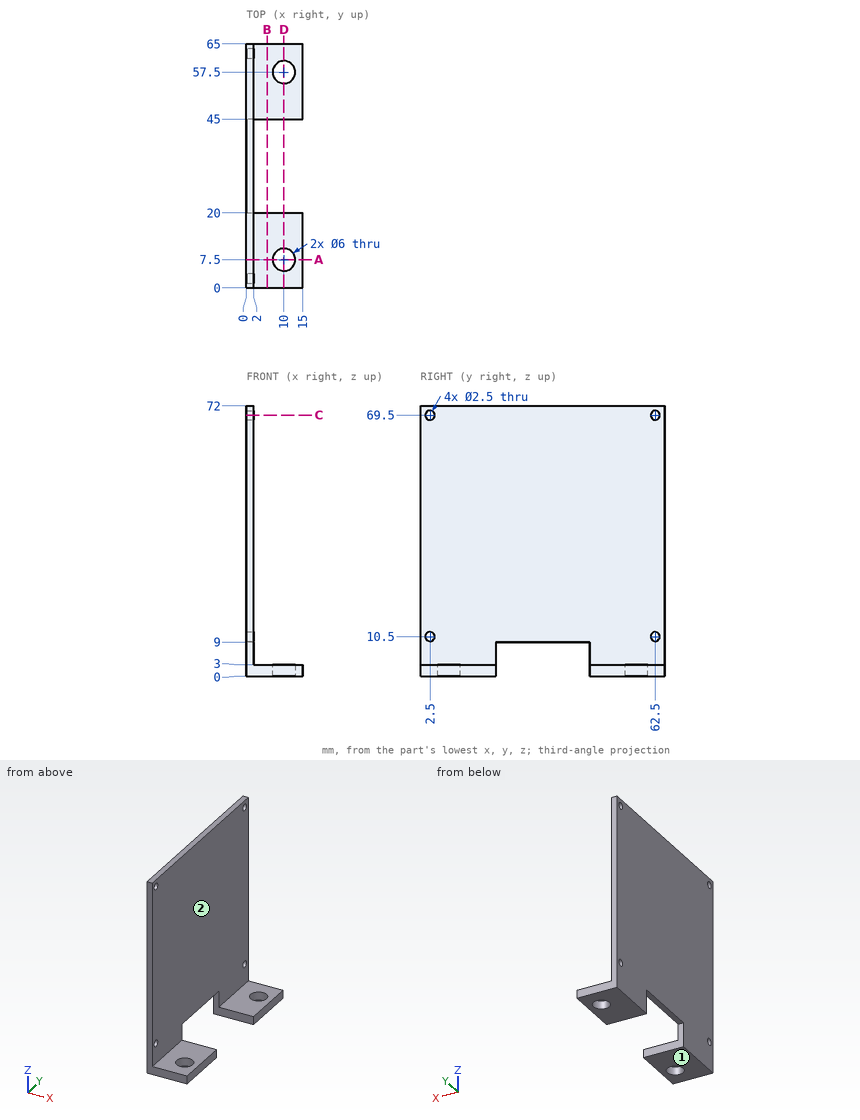
Job drawing, mm, ordinate dimensions from the low corner. One solid piece. A direction names the side the tool comes from. Round coordinates to 2 decimals unless told otherwise and drop trailing zeros. Write each loop counter-clockwise with the first axis right and the second up, starting at its lowest first coordinate (ties: lowest second). Pieces come first, ordered by that corner, then holes. Notation, with made-up numbers: (7.25, 76.5) -> (17.25, 76.5) arc R15 ccw to (17.25, 94.5) -> close; hole circle Ø9 at (-6.5, 23.25). An arc over 180 degrees is marked (long way). Answer as CSV lines item,"result".
1. Slice it at C-C, the plane z = 69.5. List the corners of the cut face in (x, y), plus the area to 3 significant figures.
Resolved:
outline,"(0, 0) -> (2, 0) -> (2, 1.25) -> (0, 1.25) -> close; (0, 3.75) -> (2, 3.75) -> (2, 61.25) -> (0, 61.25) -> close; (0, 63.75) -> (2, 63.75) -> (2, 65) -> (0, 65) -> close"
area,"120 mm²"
2. Slice it at A-A, the plane y = 7.5. List the corners of the cut face in (x, z), plus the area to 3 significant figures.
Resolved:
outline,"(0, 0) -> (7, 0) -> (7, 3) -> (2, 3) -> (2, 72) -> (0, 72) -> close; (13, 0) -> (15, 0) -> (15, 3) -> (13, 3) -> close"
area,"165 mm²"
3. Pin check, flat tips, straight feed: pin 1 Ø6.5 at (x, y) = (11.5, 13.5) entering from +Z; pin 2 Ø1 at (x, y) = (1.5, 34) entering from -Z; pin 3 Ø1.5 at (y, z) = (56.5, 23) entering from +X; pin 4 Ø7 at (x, z) = (8.5, 5) entering from +Y. Stop position of each tip, or through.
Resolved:
pin 1,"z = 3"
pin 2,"z = 9"
pin 3,"x = 2"
pin 4,"y = 65"
4. Slice it at D-D, the plane x = 10. List the corners of the cut face in (y, z), plus the area to 3 significant figures.
Resolved:
outline,"(0, 0) -> (4.5, 0) -> (4.5, 3) -> (0, 3) -> close; (10.5, 0) -> (20, 0) -> (20, 3) -> (10.5, 3) -> close; (45, 0) -> (54.5, 0) -> (54.5, 3) -> (45, 3) -> close; (60.5, 0) -> (65, 0) -> (65, 3) -> (60.5, 3) -> close"
area,"84.0 mm²"
5. Tool access for the marked faces 1 and 2: list every direction of +Z, -Z, +X, -X, +Y, -Y with a clear straight run to the whole face (end or side of a thin tool).
Resolved:
face 1,"-Z, +X, -X, +Y, -Y"
face 2,"+Z, +X, +Y, -Y"
6. Drill centre lines: line 1 (Z direction, x = 1.4, y = 2.5); line 2 (Y direction, x = 10, z = 1.75); line 3 (Y direction, x = 1.15, z = 69.5). Where is each one in solid material? Low to high.
Resolved:
line 1,"0 to 9.25, 11.75 to 68.25, 70.75 to 72"
line 2,"0 to 4.5, 10.5 to 20, 45 to 54.5, 60.5 to 65"
line 3,"0 to 1.25, 3.75 to 61.25, 63.75 to 65"
7. Slice it at B-B, the plane x = 5.5. List the corners of the cut face in (y, z).
Resolved:
outline,"(0, 0) -> (20, 0) -> (20, 3) -> (0, 3) -> close; (45, 0) -> (65, 0) -> (65, 3) -> (45, 3) -> close"
